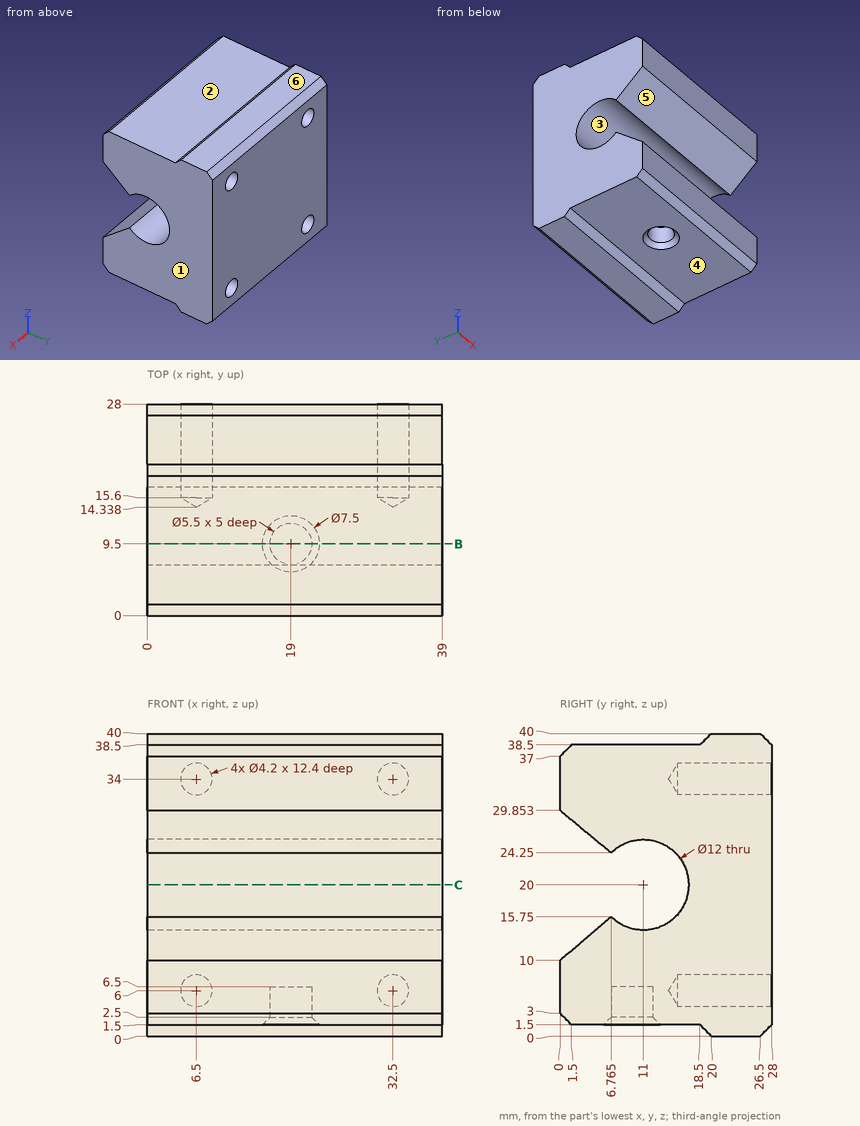
The figure shows three views and two pictorial views of one solid part (mm, origin at its lowest corner). Answer the questions. A direction names the side the tool comes from. Give positions to 0.01 mm unless a question says otherwise; leave off trailing zeros. Order: outer loops, then holes, each group sorted by start corner. A loop starts at its lowest first (then second) coordinate and runs counter-clockwise, first axis right, second up. Notation, with made-up numbers: (18, 5) -> (25, 5) arc R18 cw to (25, 39) -> close; hole circle Ø9 at (-23, 23). An arc over 180 degrees is marked (long way). Answer as CSV lines item,"result". Start each with the question number.
(1) For a pull along Z with two mould halves and no side action, classify the marked faces 1, 2 and 3 as released by +Z, released by -Z, zero draft, split by the parting line, or undercut.
(2) Which of the six approach directions +Z, -Z, +X, -X, +Y, -Y give full straight-line access (tool end or side, diameter ignored) to the marked faces 4, 5 and 6?
(3) Section C-C, the plane z = 20 is taken. Write down the section's boundary in (x, y), plus the area to 3 significant figures.
(4) Section B-B, the plane y = 9.5 is taken. Write down the section's boundary in (x, z).
(5) Consider line 1 along Z through (x, y) = (32.5, 23); line 2 along X through (y, z) = (24, 6); line 3 along Z through (x, y) = (32.5, 18.5). Determine where each line is inside the solid, lowest interval first.
(6) Each of these flat-tipped pins is pushed along its axis until it touches: pin 1 Ø1.5 at (x, z) = (24, 12.5) entering from -Y; pin 2 Ø4.5 at (x, y) = (19, 9.5) entering from -Z; pin 3 Ø3 at (x, y) = (27, 15) entering from -Z. Where does it stop, or does it pass through?
Entries:
1,face 1,"zero draft"
1,face 2,"released by +Z"
1,face 3,"undercut"
2,face 4,"-Z, +X, -X, -Y"
2,face 5,"+X, -X, -Y"
2,face 6,"+Z, +X, -X, +Y, -Y"
3,outline,"(0, 17) -> (39, 17) -> (39, 28) -> (0, 28) -> close"
3,area,"429 mm²"
4,outline,"(0, 1.5) -> (15.25, 1.5) -> (16.25, 2.5) -> (16.25, 6.5) -> (21.75, 6.5) -> (21.75, 2.5) -> (22.75, 1.5) -> (39, 1.5) -> (39, 14.19) -> (0, 14.19) -> close; (0, 25.81) -> (39, 25.81) -> (39, 38.5) -> (0, 38.5) -> close"
5,line 1,"0 to 3.9, 8.1 to 31.9, 36.1 to 40"
5,line 2,"0 to 4.4, 8.6 to 30.4, 34.6 to 39"
5,line 3,"1.5 to 3.9, 8.1 to 31.9, 36.1 to 38.5"
6,pin 1,"y = 2.06"
6,pin 2,"z = 6.5"
6,pin 3,"z = 1.5"
